Can you work these out from the model? Positions are in its coordinate system, mm. A direction names the side the tool comes from. Round coordinates to 2 decimals unless told otherwise and drop trailing zeros. Write each loop counter-clockwise with the first axis right and the second up, starting at its lowest first coordinate (ties: lowest second). Pieces come first, ordered by that corner, then holes. Notation, with made-up numbers: (26, 11.25) -> (60, 11.25) arc R21 ccw to (60, 20.25) -> close; hole circle Ø9 at (57, -9.5). An arc over 180 degrees is marked (long way). Write item = value, one per line. Start each with the question number.
1) Imagine slicing it at C-C, the plane x = 11.5. Please give me the cut outline in (y, z), then the cut area to 3 significant figures.
2) Imagine slicing it at A-A, the plane z = -32.89. Please give me the cut outline in (x, y).
3) Imagine slicing it at D-D, the plane y = 4.25. Please give me the cut outline in (x, z).
4) Thinking about a two-plate mould opening in Z: for faces 4 (the face through (40, 1, -27.32)), 5 (the face through (37.63, 4.23, -6.79)), 6 (the face through (9, 1, -5)), 7 (the face through (38.844, 3.774, -33.345)), which applies, +Z half, -Z half, draft (parallel to the pull), parting line (faces both ways), or undercut?
5) I'm going to push flat-ended pins straight in: pin 1 (1.6 mm diameter, centred on y = 1, z = -30.5, fed in from -X); pin 2 (4.5 mm diameter, centred on x = 39.5, z = -32.5, fed in from -Y); pin 3 (1 mm diameter, centred on x = 41, y = 0.5, fed in from -Z). Where does each tip first touch, or does it pass through?
6) For faces 1 (the face through (5.4, 2, -31.8)), 2 (the face through (6.79, 4.23, -6.82)), 3 (the face through (5.44, 2, -4.44)), which set-ups out of +Z, -Z, +X, -X, +Y, -Y let a thin tool reach every point of the face, with its end or its side?
7) Imagine slicing it at B-B, the plane z = -26.5. Please give me the cut outline in (x, y).
8) If I drill on line 1 (X direction, y = 2.75, z = -32.89); line 2 (Z direction, x = 41, y = 3.4); line 3 (Z direction, x = 16, y = 4.3), over which ranges is the centre line in solid material (lowest first)?
from build123d import *

# Parameters (mm, degrees)
SKETCH_1_W          = 44.45
SKETCH_1_H          = 36.32
EXTRUDE_1_DEPTH     = 5.5
SKETCH_2_R          = 2.1
CUT_EXTRUDE_1_DEPTH = 58.664502946
FILLET_2_R          = 2
CUT_EXTRUDE_START   = -5.5
SKETCH_5_W          = 32.01
SKETCH_5_H          = 23.88
CUT_EXTRUDE_2_DEPTH = 2.5
FILLET_3_R          = 2
SKETCH_6_W          = 9
SKETCH_6_H          = 9
CUT_EXTRUDE_3_DEPTH = 2


with BuildPart() as part:
    # Эскиз1 → Бобышка-Вытянуть1 (new body)
    with BuildSketch(Plane(origin=(0, 0, 0), x_dir=(1, 0, 0), z_dir=(0, 1, 0))):
        with Locations((22.225, 18.16)):
            Rectangle(SKETCH_1_W, SKETCH_1_H)
    extrude(amount=EXTRUDE_1_DEPTH)

    # Эскиз2 → Вырез-Вытянуть1 (cut, through all)
    with BuildSketch(Plane(origin=(0, 5.5, 0), x_dir=(1, 0, 0), z_dir=(0, 1, 0))):
        with Locations(Location((3.302, 32.891, 0), (0, 0, 270))):
            Circle(SKETCH_2_R)
        with Locations(Location((40.894, 32.89, 0), (0, 0, 270))):
            Circle(SKETCH_2_R)
        with Locations(Location((40.894, 3.683, 0), (0, 0, 270))):
            Circle(SKETCH_2_R)
        with Locations(Location((3.302, 3.683, 0), (0, 0, 270))):
            Circle(SKETCH_2_R)
    extrude(amount=-CUT_EXTRUDE_1_DEPTH, mode=Mode.SUBTRACT)

    # Скругление2
    fillet_2_edges = [part.edges().sort_by_distance(p)[0] for p in [
        (0, 2.75, -36.32),
        (44.45, 2.75, -36.32),
        (44.45, 2.75, 0),
        (0, 2.75, 0),
    ]]
    fillet(fillet_2_edges, radius=FILLET_2_R)

    # Эскиз5 → Вырез-Вытянуть2 (cut)
    with BuildSketch(Plane.XZ.offset(CUT_EXTRUDE_START)):
        with Locations((22.225, -18.16)):
            Rectangle(SKETCH_5_W, SKETCH_5_H)
    extrude(amount=CUT_EXTRUDE_2_DEPTH, mode=Mode.SUBTRACT)

    # Скругление3
    fillet_3_edges = [part.edges().sort_by_distance(p)[0] for p in [
        (6.22, 4.25, -30.1),
        (38.23, 4.25, -30.1),
        (38.23, 4.25, -6.22),
        (6.22, 4.25, -6.22),
    ]]
    fillet(fillet_3_edges, radius=FILLET_3_R)

    # Эскиз6 → Вырез-Вытянуть3 (cut)
    with BuildSketch(Plane.XZ):
        with Locations((4.5, -4.5)):
            Rectangle(SKETCH_6_W, SKETCH_6_H)
        with Locations((39.95, -4.5)):
            Rectangle(SKETCH_6_W, SKETCH_6_H)
        with Locations((39.95, -31.82)):
            Rectangle(SKETCH_6_W, SKETCH_6_H)
        with Locations((4.5, -31.82)):
            Rectangle(SKETCH_6_W, SKETCH_6_H)
    extrude(amount=-CUT_EXTRUDE_3_DEPTH, mode=Mode.SUBTRACT)


solid = part.part
Reported:
q1.outline = (0, -36.32) -> (5.5, -36.32) -> (5.5, -30.1) -> (3, -30.1) -> (3, -6.22) -> (5.5, -6.22) -> (5.5, 0) -> (0, 0) -> close
q1.area = 140 mm²
q2.outline = (0, 2) -> (1.2, 2) -> (1.2, 5.5) -> (0, 5.5) -> close; (5.4, 2) -> (9, 2) -> (9, 0) -> (35.45, 0) -> (35.45, 2) -> (38.79, 2) -> (38.79, 5.5) -> (5.4, 5.5) -> close; (42.99, 2) -> (44.45, 2) -> (44.45, 5.5) -> (42.99, 5.5) -> close
q3.outline = (0, -34.32) arc R2 ccw to (2, -36.32) -> (42.45, -36.32) arc R2 ccw to (44.45, -34.32) -> (44.45, -2) arc R2 ccw to (42.45, 0) -> (2, 0) arc R2 ccw to (0, -2) -> close; hole circle Ø4.2 at (3.3, -32.89); hole circle Ø4.2 at (3.3, -3.68); hole (6.22, -28.1) arc R2 ccw to (8.22, -30.1) -> (36.23, -30.1) arc R2 ccw to (38.23, -28.1) -> (38.23, -8.22) arc R2 ccw to (36.23, -6.22) -> (8.22, -6.22) arc R2 ccw to (6.22, -8.22) -> close; hole circle Ø4.2 at (40.89, -32.89); hole circle Ø4.2 at (40.89, -3.68)
q4.face_4 = -Z half
q4.face_5 = undercut
q4.face_6 = draft
q4.face_7 = undercut
q5.pin_1 = 9
q5.pin_2 = 2
q5.pin_3 = -27.32
q6.face_1 = -Z, -X, -Y
q6.face_2 = +Y
q6.face_3 = +Z, -X, -Y
q7.outline = (0, 0) -> (44.45, 0) -> (44.45, 5.5) -> (38.23, 5.5) -> (38.23, 3) -> (6.22, 3) -> (6.22, 5.5) -> (0, 5.5) -> close
q8.line_1 = 0 to 1.2, 5.4 to 38.79, 42.99 to 44.45
q8.line_2 = -36.32 to -34.99, -30.79 to -5.78, -1.59 to 0
q8.line_3 = -36.32 to -30.1, -6.22 to 0
